Source: three-view drawing plus pictorial views. Frame: mm from the lowest corner of the part. A direction names the side the tool comes from. Round coordinates to 2 decimals unless told otherwise and drop trailing zeros. Write each loop counter-clockwise with the first axis right and the second up, starting at its lowest first coordinate (ties: lowest second). Pieces come first, ordered by that corner, then holes.
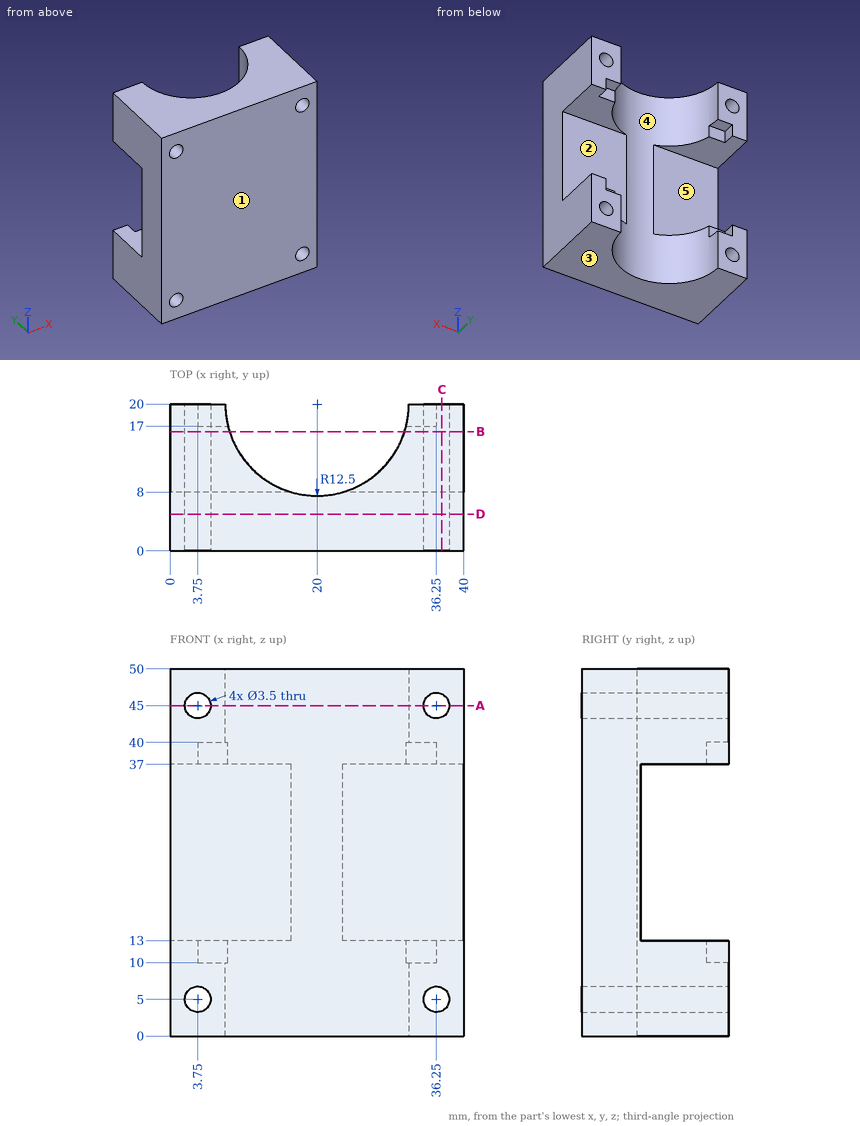
1) Line query: probe 1 along Z at (x, y) = (36.25, 13.75); probe 2 along X at (y, z) = (4.75, 5); probe 3 along Z at (x, y) = (32, 9). Output: solid intervals per line, ascending.
2) Reachability of the marked faces 4 and 5 from +Z, -Z, +X, -X, +Y, -Y: full face, straight path, thin tool, end or side. Return the list, or none.
3) Draft query along Z for the marked faces 1, 2 and 3. Return one class per face: pulls with the +Z half, pulls with the -Z half, needs draft (parallel to the pull), parting line crosses it, or undercut.
4) Section B-B on y = 16.25. Output: boundary loops of the cut face in (x, z).
5) Section A-A on z = 45. Output: boundary loops of the cut face in (x, y).
6) Section D-D on y = 5. Output: boundary loops of the cut face in (x, z), plus the area to 3 significant figures.
7) First-contact query: P1, Ø8, axis at x = 14, z = 11.5, coming from the -Y side; P2, Ø3, axis at x = 3.75, z = 45, coming from the -Y side; P3, Ø18, axis at x = 9, z = 28.5, coming from the +Y side; P4, Ø8, axis at x = 33, z = 20.5, coming from the +Y side. Flat tips, straight axial feed; report the tip coordinate or a pass-through.
8) Section C-C on x = 37. Output: boundary loops of the cut face in (y, z).
Filled in:
1. probe 1: z = 0 to 3.25, 6.75 to 13, 37 to 43.25, 46.75 to 50
1. probe 2: x = 0 to 2, 5.5 to 34.5, 38 to 40
1. probe 3: z = 0 to 13, 37 to 50
2. face 4: +Z, -Z, +Y
2. face 5: +X, -X, +Y
3. face 1: needs draft
3. face 2: undercut
3. face 3: pulls with the -Z half
4. outline: (0, 0) - (8.08, 0) - (8.08, 13) - (0, 13) - close; (0, 37) - (8.08, 37) - (8.08, 50) - (0, 50) - close; (31.92, 0) - (40, 0) - (40, 13) - (31.92, 13) - close; (31.92, 37) - (40, 37) - (40, 50) - (31.92, 50) - close; hole circle Ø3.5 at (3.75, 5); hole circle Ø3.5 at (3.75, 45); hole circle Ø3.5 at (36.25, 5); hole circle Ø3.5 at (36.25, 45)
5. outline: (0, 0) - (2, 0) - (2, 20) - (0, 20) - close; (5.5, 0) - (34.5, 0) - (34.5, 20) - (32.5, 20) arc R12.5 cw to (7.5, 20) - (5.5, 20) - close; (38, 0) - (40, 0) - (40, 20) - (38, 20) - close
6. outline: (0, 0) - (40, 0) - (40, 50) - (0, 50) - close; hole circle Ø3.5 at (3.75, 5); hole circle Ø3.5 at (3.75, 45); hole circle Ø3.5 at (36.25, 5); hole circle Ø3.5 at (36.25, 45)
6. area: 1,960 mm2
7. P1: stops at y = 0
7. P2: passes through
7. P3: stops at y = 17
7. P4: stops at y = 8
8. outline: (0, 0) - (20, 0) - (20, 3.42) - (0, 3.42) - close; (0, 6.58) - (20, 6.58) - (20, 13) - (8, 13) - (8, 37) - (20, 37) - (20, 43.42) - (0, 43.42) - close; (0, 46.58) - (20, 46.58) - (20, 50) - (0, 50) - close
